Could you check a few things on this model? Use its own coordinates, in mm. A direction names the side the tool comes from. Coordinates: 2 decimals unless noted, no trailing zeros. Order: outer loops, then holes, each group sorted by start corner. A loop starts at its lowest first (then second) coordinate and runs counter-clockwise, first axis right, second up. Notation, with made-up numbers: (18, -18) - (22, -18) arc R22 cw to (22, 16) - close; hole circle Ø4 at (-29, 11.25). An arc over 180 degrees is marked (long way). One line per item, written item: value.
from build123d import *

# Parameters (mm, degrees)
SKETCH1_R           = 2.5527
SKETCH1_R_2         = 1.905
BOSS_EXTRUDE1_DEPTH = 1.143
SKETCH3_R           = 1.905
CUT_EXTRUDE1_DEPTH  = 135.670161968
SKETCH4_W           = 50.8
SKETCH4_H           = 19.05
BOSS_EXTRUDE2_DEPTH = 2.286


with BuildPart() as part:
    # Sketch1 → Boss-Extrude1 (new, symmetric)
    with BuildSketch(Plane(origin=(0, 0, 0), x_dir=(1, 0, 0), z_dir=(0, 1, 0))):
        Polygon((-45.965990991, 39.701801802), (33.409009009, 39.701801802), (33.409009009, -49.198198198), (8.009009009, -49.198198198), (-45.965990991, 14.301801802), align=None)
        with Locations(Location((23.884009009, -33.958198198, 0), (0, 0, 270))):
            Circle(SKETCH1_R, mode=Mode.SUBTRACT)
        with Locations(Location((23.884009009, 27.001801802, 0), (0, 0, 270))):
            Circle(SKETCH1_R_2, mode=Mode.SUBTRACT)
    boss_extrude1 = extrude(amount=BOSS_EXTRUDE1_DEPTH, both=True)

    # Mirror1: Boss-Extrude1 across plane
    add(boss_extrude1.mirror(Plane(origin=(-45.965990991, 1.143, 0), x_dir=(0, 0, 1), z_dir=(-1, 0, 0))))

    # Sketch3 → Cut-Extrude1 (cut, through all)
    with BuildSketch(Plane(origin=(0, 1.143, 0), x_dir=(1, 0, 0), z_dir=(0, 1, 0))):
        with Locations(Location((-45.965990991, 27.001801802, 0), (0, 0, 270))):
            Circle(SKETCH3_R)
    extrude(amount=-CUT_EXTRUDE1_DEPTH, mode=Mode.SUBTRACT)

    # Sketch4 → Boss-Extrude2 (add)
    with BuildSketch(Plane(origin=(0, 1.143, 0), x_dir=(1, 0, 0), z_dir=(0, 1, 0))):
        with Locations((-45.965990991, 4.776801802)):
            Rectangle(SKETCH4_W, SKETCH4_H)
    extrude(amount=-BOSS_EXTRUDE2_DEPTH)


solid = part.part
Item 1: For faces 4 (the face through (-47, 1.143, -6)), 5 (the face through (-10.62, 0.02, 27.28)), which set-ups out of +Z, -Z, +X, -X, +Y, -Y let a thin tool reach every point of the face, with its end or its side?
Conclusion:
face 4: +Z, -Z, +X, -X, +Y
face 5: +Z, +Y, -Y
Item 2: If I drill on probe 1 along X at (y, z) = (-0.2, -27); probe 2 along X at (y, z) = (0.4, -26); probe 3 along Z at (x, y) = (25, 0), over which ranges is the centre line in solid material (lowest first)?
Conclusion:
probe 1: -125.34 to -117.72, -113.91 to -47.87, -44.06 to 21.98, 25.79 to 33.41
probe 2: -125.34 to -117.44, -114.2 to -47.59, -44.35 to 22.26, 25.5 to 33.41
probe 3: -39.7 to -28.55, -25.46 to 31.66, 36.25 to 49.2
Item 3: Thinking about a two-plate mould opening in X: for faces 1 (the face through (-81.31, 0.02, 27.28)), 2 (the face through (-47.13, 0.02, -28.51)), 3 (the face through (-47, -1.143, -6)), which applies, pulls with the +X half, pulls with the -X half, needs draft (parallel to the pull), parting line crosses it, or undercut?
Conclusion:
face 1: undercut
face 2: undercut
face 3: needs draft
Item 4: I want a section at B-B on y = -0.4. Please give me the cut outline in (x, z) (1 decimal), then the cut area to 3 significant figures.
Conclusion:
outline: (-125.3, -39.7) - (33.4, -39.7) - (33.4, 49.2) - (8, 49.2) - (-29.8, 4.7) - (-62.2, 4.7) - (-99.9, 49.2) - (-125.3, 49.2) - close; hole circle Ø5.1 at (-115.8, 34); hole circle Ø3.8 at (-115.8, -27); hole circle Ø3.8 at (-46, -27); hole circle Ø5.1 at (23.9, 34); hole circle Ø3.8 at (23.9, -27)
area: 10,900 mm²
Item 5: I want a section at D-D on x = -32.5. Please give me the cut outline in (y, z), then the cut area to 3 significant figures.
Conclusion:
outline: (-1.14, -39.7) - (1.14, -39.7) - (1.14, 4.75) - (-1.14, 4.75) - close
area: 102 mm²
Item 6: I'm going to push flat-ended pins straight in: pin 1 Ø1 at (x, y) = (-67.5, -1) entering from +Z; pin 2 Ø1.1 at (x, y) = (-52.5, 0) entering from +Z. Where does each tip first touch, or does it pass through?
Conclusion:
pin 1: z = 11.62
pin 2: z = 4.75
Item 7: I want a section at C-C on z = 12.5. Please give me the cut outline in (x, y), then the cut area to 3 significant figures.
Conclusion:
outline: (-125.34, -1.14) - (-68.75, -1.14) - (-68.75, 1.14) - (-125.34, 1.14) - close; (-23.18, -1.14) - (33.41, -1.14) - (33.41, 1.14) - (-23.18, 1.14) - close
area: 259 mm²
Item 8: I want a section at A-A on z = -27. Please give me the cut outline in (x, y).
Conclusion:
outline: (-125.34, -1.14) - (-117.72, -1.14) - (-117.72, 1.14) - (-125.34, 1.14) - close; (-113.91, -1.14) - (-47.87, -1.14) - (-47.87, 1.14) - (-113.91, 1.14) - close; (-44.06, -1.14) - (21.98, -1.14) - (21.98, 1.14) - (-44.06, 1.14) - close; (25.79, -1.14) - (33.41, -1.14) - (33.41, 1.14) - (25.79, 1.14) - close
